Verification items for the finished model (mm, model axes). Face numbers are marked on the shaded views. A direction names the side the tool comes from. Round coordinates to 2 decimals unless told otherwise and drop trailing zeros. Write each loop counter-clockwise with the first axis right and the second up, starting at its lowest first coordinate (ties: lowest second). Pieces come first, ordered by that corner, then holes. Notation, with made-up numbers: (78, 5.5) - (83, 5.5) arc R21 ccw to (83, 21.5) - close; hole circle Ø11 at (11.25, 8). An arc over 180 degrees is marked (long way). Answer as a JSON object with one key per item and string values.
```python
from build123d import *


with BuildPart() as part:
    # Sketch1 → Revolve1 (revolve)
    with BuildSketch(Plane.XY, mode=Mode.PRIVATE) as revolve1_sk:
        with BuildLine():
            Line((0, 0), (0, 18))
            Line((0, 18), (10, 18))
            Line((10, 18), (10, 8.5))
            ThreePointArc((10, 8.5), (10.292893219, 7.792893219), (11, 7.5))
            Line((11, 7.5), (12, 7.5))
            Line((12, 7.5), (12, 6.2))
            ThreePointArc((12, 6.2), (12.058578644, 6.058578644), (12.2, 6))
            Line((12.2, 6), (32, 6))
            Line((32, 6), (32, 0))
            Line((32, 0), (0, 0))
        make_face()
    revolve(revolve1_sk.sketch.rotate(Axis((32, 0, 0), (-1, 0, 0)), 270), axis=Axis((32, 0, 0), (-1, 0, 0)))

    # Sketch2 → Cut-Revolve1 (revolve, cut)
    with BuildSketch(Plane.XY, mode=Mode.PRIVATE) as cut_revolve1_sk:
        Polygon((0, 13), (0, 15.5), (0.433, 15.067), (5.167, 15.067), (5.6, 15.5), (5.6, 17), (10, 17), (10, 13), align=None)
    revolve(cut_revolve1_sk.sketch.rotate(Axis((10, 13, 0), (-1, 0, 0)), 270), axis=Axis((10, 13, 0), (-1, 0, 0)), mode=Mode.SUBTRACT)

    # Sketch3 → Cut-Revolve2 (revolve, cut)
    with BuildSketch(Plane.XY.offset(13), mode=Mode.PRIVATE) as cut_revolve2_sk:
        Polygon((0, 0), (0, 2.5), (0.433, 2.067), (5.167, 2.067), (5.6, 2.5), (5.6, 4), (10, 4), (10, 0), align=None)
    revolve(cut_revolve2_sk.sketch.rotate(Axis((10, 0, 13), (-1, 0, 0)), 270), axis=Axis((10, 0, 13), (-1, 0, 0)), mode=Mode.SUBTRACT)

    # Sketch4 → Cut-Revolve3 (revolve, cut)
    with BuildSketch(Plane.XY, mode=Mode.PRIVATE) as cut_revolve3_sk:
        Polygon((0, -13), (0, -10.5), (0.433, -10.933), (5.167, -10.933), (5.6, -10.5), (5.6, -9), (10, -9), (10, -13), align=None)
    revolve(cut_revolve3_sk.sketch.rotate(Axis((10, -13, 0), (-1, 0, 0)), 270), axis=Axis((10, -13, 0), (-1, 0, 0)), mode=Mode.SUBTRACT)

    # Sketch5 → Cut-Revolve4 (revolve, cut)
    with BuildSketch(Plane.XY.offset(-13), mode=Mode.PRIVATE) as cut_revolve4_sk:
        Polygon((0, 0), (0, 2.5), (0.433, 2.067), (5.167, 2.067), (5.6, 2.5), (5.6, 4), (10, 4), (10, 0), align=None)
    revolve(cut_revolve4_sk.sketch.rotate(Axis((10, 0, -13), (-1, 0, 0)), 270), axis=Axis((10, 0, -13), (-1, 0, 0)), mode=Mode.SUBTRACT)

    # Sketch6 → Cut-Revolve5 (revolve, cut)
    with BuildSketch(Plane.XY, mode=Mode.PRIVATE) as cut_revolve5_sk:
        Polygon((7, 0), (8.91882362, 3.3235), (31.3235, 3.3235), (32, 4), (32, 0), align=None)
    revolve(cut_revolve5_sk.sketch.rotate(Axis((32, 0, 0), (-1, 0, 0)), 270), axis=Axis((32, 0, 0), (-1, 0, 0)), mode=Mode.SUBTRACT)


solid = part.part
```
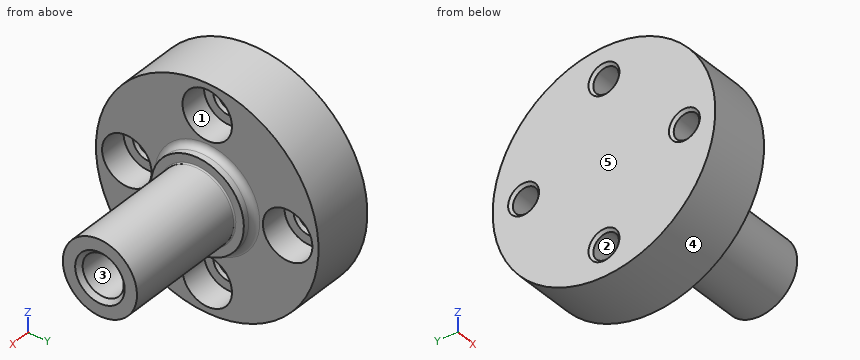
1. Cross-section at B-B (x = 16). Record the boundary of the cut face in (y, z).
Completed:
{"outline": "circle Ø12 at (0, 0); hole circle Ø6.65 at (0, 0)"}
2. Cross-section at D-D (x = 11.5). Record the boundary of the cut face in (y, z), plus the area to 3 significant figures.
Completed:
{"outline": "circle Ø15 at (0, 0); hole circle Ø6.65 at (0, 0)", "area": "142 mm^2"}
3. Cross-section at A-A (y = -13). Record the boundary of the cut face in (x, z).
Completed:
{"outline": "(0, -12.45) - (10, -12.45) - (10, -4) - (5.6, -4) - (5.6, -2.5) - (5.17, -2.07) - (0.43, -2.07) - (0, -2.5) - close; (0, 2.5) - (0.43, 2.07) - (5.17, 2.07) - (5.6, 2.5) - (5.6, 4) - (10, 4) - (10, 12.45) - (0, 12.45) - close"}
4. Go/stop test with flat-tipped pins: pin 1 (1 mm diameter, centred on x = 10, z = 11.5, fed in from -Y); pin 2 (5 mm diameter, centred on x = 21, z = -7.5, fed in from +Y); pin 3 (3.5 mm diameter, centred on y = 0, z = 13, fed in from -X); pin 4 (3 mm diameter, centred on x = 4.5, z = 11, fed in from -Y). Record where each tip stops, or that it passes through.
Completed:
{"pin 1": "stops at y = -14.25", "pin 2": "stops at y = 3.32", "pin 3": "passes through", "pin 4": "stops at y = -15.29"}
5. Material ranges on probe 1 along Y at (x, z) = (3, 0); probe 2 along Y at (x, z) = (26, 0); probe 3 along Y at (x, z) = (7.3, 0), recorded low to high. Write a range as from..to.
Completed:
{"probe 1": "y = -18..-15.07, -10.93..10.93, 15.07..18", "probe 2": "y = -6..-3.32, 3.32..6", "probe 3": "y = -18..-17, -9..-0.52, 0.52..9, 17..18"}
6. Mould release check, pull along Y, two halves, no side actions. Record for the marked faces 3, 4 and 5: released by +Y, released by -Y, zero draft, split by the parting line, or undercut.
Completed:
{"face 3": "undercut", "face 4": "split by the parting line", "face 5": "zero draft"}
7. Access from +Z, -Z, +X, -X, +Y, -Y to the whole of each face (thin tool, end or side, straight path). Record for the marked faces 1 and 2.
Completed:
{"face 1": "+X", "face 2": "+X, -X"}
